```python
from build123d import *

# Parameters (mm, degrees)
SKETCH_1_R          = 5
EXTRUDE_1_DEPTH     = 3
SKETCH_2_R          = 2.5
CUT_EXTRUDE_1_DEPTH = 131.896905999
EXTRUDE_START       = -3
SKETCH_3_R          = 5
EXTRUDE_2_DEPTH     = 3
SKETCH_4_R          = 1.5
CUT_EXTRUDE_2_DEPTH = 3
SKETCH_5_W          = 5
SKETCH_5_H          = 5.5
SKETCH_5_W_2        = 5.5
SKETCH_5_H_2        = 5
SKETCH_5_R          = 1.5
CUT_EXTRUDE_3_DEPTH = 2


with BuildPart() as part:
    # 草图1 → 凸台-拉伸1 (new body)
    with BuildSketch(Plane(origin=(0, 0, 0), x_dir=(1, 0, 0), z_dir=(0, 1, 0))):
        with BuildLine():
            Line((0, -15), (120.415586748, -9.991360651))
            ThreePointArc((120.415586748, -9.991360651), (130, 0), (120.415586748, 9.991360651))
            Line((120.415586748, 9.991360651), (0, 15))
            ThreePointArc((0, 15), (-15, 0), (0, -15))
        make_face()
        with Locations(Location((0, 0, 0), (0, 0, 270))):
            Circle(SKETCH_1_R, mode=Mode.SUBTRACT)
    extrude(amount=EXTRUDE_1_DEPTH)

    # 草图2 → 切除-拉伸1 (cut, through all)
    with BuildSketch(Plane(origin=(0, 3, 0), x_dir=(1, 0, 0), z_dir=(0, 1, 0))):
        with Locations(Location((120, 0, 0), (0, 0, 270))):
            Circle(SKETCH_2_R)
    extrude(amount=-CUT_EXTRUDE_1_DEPTH, mode=Mode.SUBTRACT)

    # 草图3 → 凸台-拉伸2 (add)
    with BuildSketch(Plane(origin=(0, 3, 0), x_dir=(1, 0, 0), z_dir=(0, 1, 0)).offset(EXTRUDE_START)):
        Circle(SKETCH_3_R)
    extrude(amount=EXTRUDE_2_DEPTH)

    # 草图4 → 切除-拉伸2 (cut)
    with BuildSketch(Plane(origin=(0, 3, 0), x_dir=(1, 0, 0), z_dir=(0, 1, 0))):
        with Locations(Location((0, 0, 0), (0, 0, 270))):
            Circle(SKETCH_4_R)
    extrude(amount=-CUT_EXTRUDE_2_DEPTH, mode=Mode.SUBTRACT)

    # 草图5 → 切除-拉伸3 (cut)
    # profile 1 of 5: a face of its own
    with BuildSketch(Plane(origin=(0, 3, 0), x_dir=(1, 0, 0), z_dir=(0, 1, 0))):
        with Locations((0, 5.25)):
            Rectangle(SKETCH_5_W, SKETCH_5_H)
    # profile 2 of 5: a face of its own
    with BuildSketch(Plane(origin=(0, 3, 0), x_dir=(1, 0, 0), z_dir=(0, 1, 0))):
        with Locations((-5.25, 0)):
            Rectangle(SKETCH_5_W_2, SKETCH_5_H_2)
    # profile 3 of 5: a face of its own
    with BuildSketch(Plane(origin=(0, 3, 0), x_dir=(1, 0, 0), z_dir=(0, 1, 0))):
        with Locations((0, -5.25)):
            Rectangle(SKETCH_5_W, SKETCH_5_H)
    # profile 4 of 5: a face of its own
    with BuildSketch(Plane(origin=(0, 3, 0), x_dir=(1, 0, 0), z_dir=(0, 1, 0))):
        with Locations((5.25, 0)):
            Rectangle(SKETCH_5_W_2, SKETCH_5_H_2)
    # profile 5 of 5: a face of its own
    with BuildSketch(Plane(origin=(0, 3, 0), x_dir=(1, 0, 0), z_dir=(0, 1, 0))):
        Rectangle(SKETCH_5_W, SKETCH_5_H_2)
        with Locations(Location((0, 0, 0), (0, 0, 270))):
            Circle(SKETCH_5_R, mode=Mode.SUBTRACT)
    extrude(amount=-CUT_EXTRUDE_3_DEPTH, mode=Mode.SUBTRACT)


solid = part.part
```
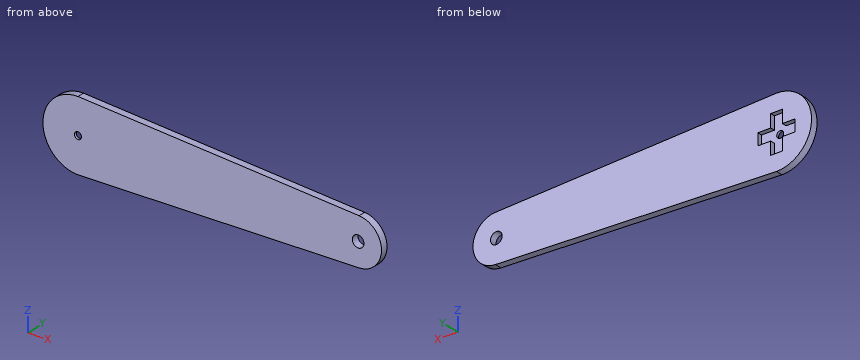
Geometry: final body of the model. Coordinates: model frame, mm. Round coordinates to 2 decimals unless told otherwise and drop trailing zeros. Order: outer loops, then holes, each group sorted by start corner. A loop starts at its lowest first (then second) coordinate and runs counter-clockwise, first axis right, second up. Notation, with made-up numbers: (-20, 31) -> (5, 31) arc R9 cw to (5, 46) -> close; hole circle Ø11 at (-9, -38). An arc over 180 degrees is marked (long way). Use one line per item in the form item = value. Start each with the question number.
1. Cut plane C-C (z = 6). Return the cut outline in (x, y).
2. Cut plane B-B (y = 1.45). Return the cut outline in (x, z).
3. Line query: probe 1 along X at (y, z) = (1.55, 0); probe 2 along X at (y, z) = (0.3, 0); probe 3 along Z at (x, y) = (119, 0.65). Output: solid intervals per line, ascending.
4. Pin query (flat end, axial travel): pin 1 Ø1 at (y, z) = (2.5, 1) entering from +X; pin 2 Ø1.6 at (x, y) = (4.5, 2) entering from +Z; pin 3 Ø0.6 at (y, z) = (2, -4) entering from +X; pin 4 Ø8 at (x, z) = (120, 0) entering from +Y. Return the tip coordinate at first contact, or that it passes through.
5. Cut plane D-D (x = 28). Return the cut outline in (y, z).
6. Cut plane A-A (z = 0). Return the cut outline in (x, y).
Solution:
q1.outline = (-13.75, 0) -> (128, 0) -> (128, 3) -> (2.5, 3) -> (2.5, 1) -> (-2.5, 1) -> (-2.5, 3) -> (-13.75, 3) -> close
q2.outline = (0, -15) -> (120.42, -9.99) arc R10 ccw to (120.42, 9.99) -> (0, 15) arc R15 ccw to start; hole (-8, -2.5) -> (-2.5, -2.5) -> (-2.5, -8) -> (2.5, -8) -> (2.5, -2.5) -> (8, -2.5) -> (8, 2.5) -> (2.5, 2.5) -> (2.5, 8) -> (-2.5, 8) -> (-2.5, 2.5) -> (-8, 2.5) -> close; hole circle Ø5 at (120, 0)
q3.probe_1 = -15 to -8, 8 to 117.5, 122.5 to 130
q3.probe_2 = -15 to -1.5, 1.5 to 117.5, 122.5 to 130
q3.probe_3 = -10.05 to -2.29, 2.29 to 10.05
q4.pin_1 = 129.99
q4.pin_2 = 14.85
q4.pin_3 = 129.29
q4.pin_4 = 3
q5.outline = (0, -13.84) -> (3, -13.84) -> (3, 13.84) -> (0, 13.84) -> close
q6.outline = (-15, 0) -> (-1.5, 0) -> (-1.5, 1) -> (-8, 1) -> (-8, 3) -> (-15, 3) -> close; (1.5, 0) -> (117.5, 0) -> (117.5, 3) -> (8, 3) -> (8, 1) -> (1.5, 1) -> close; (122.5, 0) -> (130, 0) -> (130, 3) -> (122.5, 3) -> close
